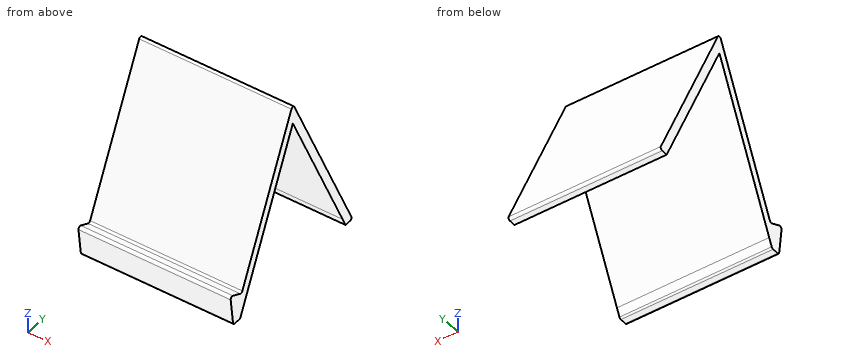
```python
from build123d import *

# Parameters (mm, degrees)
F1_DEPTH = 70
F2_R     = 1


with BuildPart() as f1:
    # F0 (on Right) → F1 (new body)
    with BuildSketch(Plane.YZ):
        Polygon((-1.8379441239, 14.9881287721), (0, 0), (4.4135116758, 0), (6.2787423085, 4), (38.0356435567, 72.1028945007), (69.7925448049, 4), (71.6577754375, 0), (76.0712871133, 0), (38.0356435567, 81.5677008333), (5.4125181724, 11.6071826782), align=None)
    extrude(amount=F1_DEPTH)

    # F2
    f2_edges = [f1.edges().sort_by_distance(p)[0] for p in [
        (35, -1.837944, 14.988129),
        (35, 5.412518, 11.607183),
        (35, 38.035644, 81.567701),
        (35, 0, 0),
        (35, 76.071287, 0),
        (35, 4.413512, 0),
    ]]
    fillet(f2_edges, radius=F2_R)


solid = f1.part
```
The listing builds one solid part. Answer for the finished solid, in the listing's coordinates (mm). Give positions to 0.01 mm unless a question says otherwise; leave off trailing zeros. Loops run counter-clockwise (first coordinate to the right, second up) from the corner with the lowest first, then second, coordinate; pieces in that order, holes last. Notation, with made-up numbers: M 61.25,-16.5 L 87.25,-16.5 A9 cw 87.25,-10.5 Z; hole C 7,-18 d9. An arc over 180 degrees is marked long. One line per item, written item: value.
Q1. A cutting plane is placed at C-C on y = 40. Determine the outline of the cut face in (x, z).
Working result:
outline: M 0,67.89 L 70,67.89 L 70,77.36 L 0,77.36 Z
Q2. A cutting plane is placed at D-D on z = 74.5. Determine the outline of the cut face in (x, y).
Working result:
outline: M 0,34.74 L 70,34.74 L 70,41.33 L 0,41.33 Z
Q3. A cutting plane is placed at A-A on x = 32. Determine the outline of the cut face in (y, z).
Working result:
outline: M -1.62,13.2 L -0.11,0.88 A1 ccw 0.88,0 L 3.78,0 A1 ccw 4.68,0.58 L 38.04,72.1 L 71.66,0 L 74.5,0 A1 ccw 75.41,1.42 L 38.94,79.62 A1 ccw 37.13,79.62 L 5.84,12.51 A1 cw 4.51,12.03 L -0.2,14.23 A1 ccw Z
Q4. Find the intervals of material crossed by line 1 (Y direction, x = 16, z = 21.5); line 2 (Y direction, x = 41, z = 7); line 3 (Z direction, x = 14, y = 69), in increasing order. Write a range as from..to.
Working result:
line 1: y = 10.03..14.44, 61.63..66.05
line 2: y = -0.86..7.68, 68.39..72.81
line 3: z = 5.7..15.16
Q5. Flat-ended cylindrical pins translate along their axes: P1, Ø2, axis at x = 46, z = 67.5, coming from the -Y side; P2, Ø10, axis at x = 35, y = 20.5, coming from the -Z side; P3, Ø3, axis at x = 23.5, z = 63.5, coming from the +Y side; P4, Ø1, axis at y = 54, z = 32, coming from the +X side. Find the tip coordinate at first contact, or state that the pin passes through.
Working result:
P1: stops at y = 31.01
P2: stops at z = 23.78
P3: stops at y = 47.16
P4: passes through
Q6. A cutting plane is placed at B-B on z = 61.5. Determine the outline of the cut face in (x, y).
Working result:
outline: M 0,28.68 L 70,28.68 L 70,33.09 L 0,33.09 Z; M 0,42.98 L 70,42.98 L 70,47.39 L 0,47.39 Z
